Input: part model. Units: mm. Frame: model coordinates. A direction names the side the tool comes from. Round coordinates to 2 decimals unless told otherwise and drop trailing zeros. Write each loop counter-clockwise with the first axis right and the second up, starting at its lowest first coordinate (ties: lowest second). Pieces come first, ordered by that corner, then holes. Notation, with made-up numbers: (79, 0) -> (98, 0) arc R27 ccw to (98, 35) -> close; hole circle Ø4 at (51.25, 76.5). An arc over 180 degrees is marked (long way). Write item = value, one per line. Start each with the question number.
Autodesk Inventor part; units mm, degrees
ref_plane "YZ Plane" through (0, 0, 0) normal (1, 0, 0) x (0, 1, 0)
ref_plane "XZ Plane" through (0, 0, 0) normal (0, 1, 0) x (-1, 0, 0)
ref_plane "XY Plane" through (0, 0, 0) normal (0, 0, 1) x (1, 0, 0)
sketch "Sketch1" plane through (0, 0, 0) normal (0, 0, 1) x (1, 0, 0)
  line L0 (-12.1245, 12.5373) -> (64.0755, 12.5373)
  line L1 (64.0755, 12.5373) -> (64.0755, -114.4627)
  line L2 (64.0755, -114.4627) -> (-12.1245, -114.4627)
  line L3 (-12.1245, -114.4627) -> (-12.1245, 12.5373)
  point P0 (0, 0)
  dimension "d0" = 76.2
  dimension "d1" = 127
extrude "Extrusion1" add sketch "Sketch1" along normal blind 6.35
sketch "Sketch2" plane through (0, 0, 6.35) normal (0, 0, 1) x (1, 0, 0)
  line L0 (-12.1245, -114.4627) -> (64.0755, -114.4627)
  line L1 (25.9755, -114.4627) -> (25.9755, 12.062) construction
  line L2 (21.4802, -114.4627) -> (21.4802, -38.2627)
  line L3 (30.4708, -114.4627) -> (30.4708, -38.2627)
  line L4 (21.4802, -38.2627) -> (30.4708, -38.2627)
  line L5 (21.4802, -114.4627) -> (30.4708, -114.4627)
  point P0 (0, 0)
  dimension "d4" = 76.2
extrude "Extrusion2" add sketch "Sketch2" along normal blind 25.4
sketch "Sketch3" plane through (0, 0, 31.75) normal (0, 0, 1) x (1, 0, 0)
  line L0 (64.0755, -114.4627) -> (64.0755, 12.5373)
  line L1 (-12.1245, -114.4627) -> (64.0755, -114.4627)
  line L2 (64.0755, -114.4627) -> (64.0755, 0)
  line L3 (64.0755, 0) -> (-12.1245, 0)
  line L4 (-12.1245, 0) -> (-12.1245, -114.4627)
  point P0 (0, 0)
extrude "Extrusion3" add sketch "Sketch3" along normal blind 6.35
sketch "Sketch4" plane through (0, 0, 31.75) normal (0, 0, -1) x (-1, 0, 0)
  point P0 (0, 0)
sketch "Sketch5" plane through (0, 0, 6.35) normal (0, 0, 1) x (1, 0, 0)
  line L0 (21.4802, -38.2627) -> (30.4708, -38.2627)
  line L1 (25.9755, -38.2627) -> (25.9755, -33.1827) construction
  circle A0 centre (25.9755, -33.1827) radius 3.175
  point P0 (0, 0)
  dimension "d9" = 5.08
  dimension "d10" = 6.35
extrude "Extrusion4" cut sketch "Sketch5" along normal mid plane 76.2
sketch "Sketch6" plane through (64.0755, -114.4627, 31.75) normal (1, 0, 0) x (0, 0, -1)
  line L0 (31.75, 127) -> (31.75, 0)
  line L1 (-6.35, 114.4627) -> (31.75, 114.4627)
  line L2 (31.75, 114.4627) -> (31.75, 0)
  line L3 (31.75, 0) -> (-6.35, 0)
  line L4 (-6.35, 0) -> (-6.35, 114.4627)
extrude "Extrusion5" add sketch "Sketch6" along normal blind 6.35
sketch "Sketch7" plane through (-12.1245, -114.4627, 31.75) normal (-1, 0, 0) x (0, 0, 1)
  line L0 (0, 114.4627) -> (6.35, 114.4627)
  line L1 (-31.75, 0) -> (-25.4, 0)
  line L2 (6.35, 114.4627) -> (-31.75, 114.4627)
  line L3 (-31.75, 114.4627) -> (-31.75, 0)
  line L4 (-31.75, 0) -> (6.35, 0)
  line L5 (6.35, 0) -> (6.35, 114.4627)
extrude "Extrusion6" add sketch "Sketch7" along normal blind 6.35
sketch "Sketch8" plane through (64.0755, 0, 31.75) normal (0, 1, 0) x (1, 0, 0)
  line L0 (-82.55, 31.75) -> (6.35, 31.75)
  line L1 (0, 0) -> (-76.2, 0)
  line L2 (-82.55, 31.75) -> (-76.2, 31.75)
  line L3 (-76.2, 31.75) -> (-76.2, 0)
  line L4 (-82.55, 0) -> (-82.55, 31.75)
  line L5 (6.35, 31.75) -> (6.35, -6.35)
  line L6 (-76.2, 0) -> (0, 0)
  line L7 (6.35, 0) -> (6.35, -6.35)
  line L8 (6.35, -6.35) -> (-82.55, -6.35)
  line L9 (-82.55, -6.35) -> (-82.55, 0)
  line L10 (0, 31.75) -> (0, 25.4)
  line L11 (0, 0) -> (0, 31.75)
  line L12 (0, 31.75) -> (6.35, 31.75)
  line L13 (6.35, 31.75) -> (6.35, 0)
  point P0 (-64.0755, 31.75)
extrude "Extrusion7" add sketch "Sketch8" along normal blind 12.7 contours L0 L3 L1 L11 L10 L5 L8 L9 L4
sketch "Sketch9" plane through (64.0755, 12.5373, 6.35) normal (0, 1, 0) x (1, 0, 0)
  line L0 (-76.2, 0) -> (-42.5953, 0)
  line L1 (-82.55, 6.35) -> (6.35, 6.35)
  line L2 (-76.2, 0) -> (0.0054, 0)
  line L3 (0.0054, 0) -> (0.0054, 6.35)
  line L4 (0.0054, 6.35) -> (-76.2, 6.35)
  line L5 (-76.2, 6.35) -> (-76.2, 0)
  point P0 (-64.0755, 6.35)
extrude "Extrusion8" add sketch "Sketch9" along normal up to surface (0.1627 mm away)
sketch "Sketch10" plane through (0, 0, 38.1) normal (0, 0, 1) x (1, 0, 0)
  line L0 (64.0755, 12.7) -> (-12.1245, 12.7) construction
  line L1 (64.0755, -114.4627) -> (64.0755, 12.7)
  line L2 (-12.1245, 12.7) -> (64.0755, 12.7) construction
  line L3 (64.0755, 12.7) -> (64.0755, -63.5) construction
  line L4 (64.0755, -63.5) -> (-12.1245, -63.5) construction
  line L5 (-12.1245, -63.5) -> (-12.1245, 12.7) construction
  line L6 (-12.1245, 12.7) -> (25.9755, -25.4)
  line L7 (64.0755, 12.7) -> (25.9755, -25.4)
  line L8 (-12.1245, -114.4627) -> (-12.1245, 12.7)
  line L9 (-12.1245, 12.7) -> (64.0755, 12.7)
  point P0 (0, 0)
  dimension "d21" = 76.2
extrude "Extrusion9" cut sketch "Sketch10" against normal blind 25.4
properties part number "ENGR131 KC Design" material "Concrete Masonry Units"
1. Line query: line 1 along X through (y, z) = (-79, 13.5); line 2 along Z through (x, y) = (6.5, -34); line 3 along X through (y, z) = (1, 23.5). Output: solid intervals per line, ascending.
2. Mould query, pull axis Z, two halves, no side actions, for faces 6 (the cylindrical face through (25.287, -30.083, 34.881)), 7 (the flat face through (35, -52, 31.75)), 8 (the flat face through (30.471, -77, 19)), 9 (the flat face through (27, -52, 38.1)). Classes: pulls with the +Z half, pulls with the -Z half, needs draft (parallel to the pull), parting line crosses it, or undercut.
3. Pin query (flat end, axial travel): P1, Ø1.5, axis at x = -5.5, z = 8.5, coming from the +Y side; P2, Ø10, axis at x = 24, z = 13, coming from the +Y side. Return the tip coordinate at first contact, or that it passes through.
4. Section B-B (y = -90.5). Output: boundary loops of the cut face in (x, z).
5. Reachability of faces 1 (the flat face through (45.292, -6.083, 34.969)), 2 (the flat face through (70.426, -50, 19)), 3 (the flat face through (26, -38.263, 19)), 4 (the flat face through (25, 12.7, 6)), 5 (the flat face through (64.076, -52, 19)) from +Z, -Z, +X, -X, +Y, -Y: full face, straight path, thin tool, end or side. Return the list, or none.
6. Section A-A (z = 8). Output: boundary loops of the cut face in (x, y), then the cut area to 3 significant figures.
7. Section C-C (x = 6). Output: boundary loops of the cut face in (y, z).
Check sheet entries:
q1.line_1 = -18.47 to -12.12, 21.48 to 30.47, 64.08 to 70.43
q1.line_2 = 0 to 6.35, 31.75 to 38.1
q1.line_3 = -18.47 to -12.12, 64.08 to 70.43
q2.face_6 = needs draft
q2.face_7 = undercut
q2.face_8 = undercut
q2.face_9 = pulls with the +Z half
q3.P1 = through
q3.P2 = -38.26
q4.outline = (-18.47, 0) -> (70.43, 0) -> (70.43, 38.1) -> (-18.47, 38.1) -> close; hole (-12.12, 6.35) -> (21.48, 6.35) -> (21.48, 31.75) -> (-12.12, 31.75) -> close; hole (30.47, 6.35) -> (64.08, 6.35) -> (64.08, 31.75) -> (30.47, 31.75) -> close
q5.face_1 = +Z, +Y
q5.face_2 = +Z, -Z, +X, +Y, -Y
q5.face_3 = +Y
q5.face_4 = +Z, -Z, +X, -X, +Y
q5.face_5 = +Y, -Y
q6.outline = (-18.47, -114.46) -> (-12.12, -114.46) -> (-12.12, 12.7) -> (-18.47, 12.7) -> close; (21.48, -114.46) -> (30.47, -114.46) -> (30.47, -38.26) -> (21.48, -38.26) -> close; (64.08, -114.46) -> (70.43, -114.46) -> (70.43, 12.7) -> (64.08, 12.7) -> close
q6.area = 2,300 mm2
q7.outline = (-114.46, 0) -> (12.7, 0) -> (12.7, 6.35) -> (-114.46, 6.35) -> close; (-114.46, 31.75) -> (-5.42, 31.75) -> (-5.42, 38.1) -> (-114.46, 38.1) -> close
